Check sheet for the modelled part. Datum: model origin and axes. Units: mm. Face numbers are marked on the shaded views. A direction names the side the tool comes from. Give positions to 0.01 mm unless a question says otherwise; leave off trailing zeros. Write each loop counter-clockwise with the first axis right and the second up, starting at its lowest first coordinate (ties: lowest second). Pieces come first, ordered by that corner, then holes. Notation, with made-up numbers: M 51,79 L 81,79 A27 cw 81,110 Z; hole C -21,-19 d8. An arc over 180 degrees is marked long. Write item = value, one per line. Start each with the question number.
1) Sectioned sample at B-B, the plane x = 153. Record the cut outline in (y, z).
2) Sectioned sample at D-D, the plane z = 280. Record the cut outline in (x, y).
3) Sectioned sample at C-C, the plane x = -87. Record the cut outline in (y, z).
4) Scan lines: L1, parallel to Z at x = -26, y = -2.5; L2, parallel to Y at x = 56, z = 376; L3, parallel to X at y = 3.5, z = -16.5. Record each from-to range of solid material in increasing order.
5) Sectioned sample at A-A, the plane z = 67. Record the cut outline in (x, y).
6) Set-up check for the marked faces 1, 2 and 3: record each of +Z, -Z, +X, -X, +Y, -Y from which the full face is reachable in a straight line by a thin tool's end or side.
7) Gauge pin test, flat ends, axial feed: pin 1 (2 mm diameter, centred on x = -150.5, y = -1, fed in from -Z); pin 2 (6 mm diameter, centred on x = 18.5, z = 249.5, fed in from +Y); pin 3 (0.8 mm diameter, centred on x = 141.5, y = -0.5, fed in from +Z). Record the tip position at first contact, or that the pin passes through.
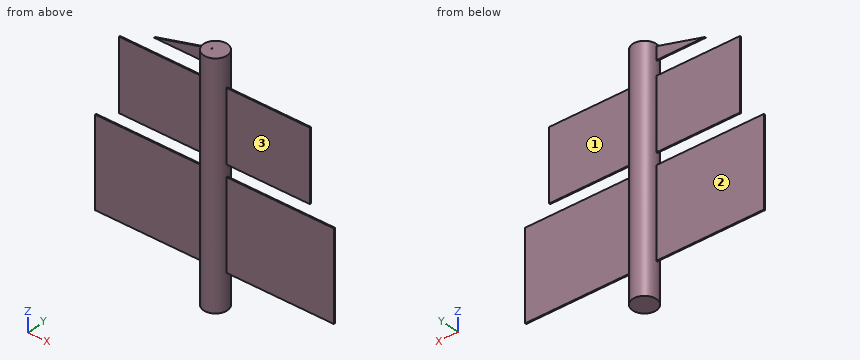
from build123d import *

# Parameters (mm, degrees)
F0_W     = 25.4
F0_H     = 508
F2_W     = 508
F2_H     = 190.5
F3_DEPTH = 2.54
F4_W     = 406.4
F4_H     = 152.4
F5_DEPTH = 2.54


with BuildPart() as f1:
    # F0 (on Front) → F1 (revolve)
    with BuildSketch(Plane.XZ):
        with Locations((12.7, 197.317208)):
            Rectangle(F0_W, F0_H)
    revolve(axis=Axis((0, 0, 197.317208), (0, 0, 1)))

    # F2 (on Front) → F3 (join)
    with BuildSketch(Plane.XZ):
        with Locations((0, 114.767208)):
            Rectangle(F2_W, F2_H)
    extrude(amount=F3_DEPTH)

    # F4 (on Front) → F5 (join)
    with BuildSketch(Plane.XZ):
        with Locations((0, 311.617208)):
            Rectangle(F4_W, F4_H)
        Polygon((-6.016195, 419.029802), (-6.016195, 452.049802), (-128.64849, 419.029802), align=None)
    extrude(amount=F5_DEPTH)


solid = f1.part
Data:
q1.outline = M -2.54,19.52 L 0,19.52 L 0,210.02 L -2.54,210.02 Z; M -2.54,235.42 L 0,235.42 L 0,387.82 L -2.54,387.82 Z
q2.outline = M -203.2,-2.54 L -25.27,-2.54 A25.4 ccw 25.27,-2.54 L 203.2,-2.54 L 203.2,0 L 25.4,0 A25.4 ccw -25.4,0 L -203.2,0 Z
q3.outline = M -2.54,19.52 L 0,19.52 L 0,210.02 L -2.54,210.02 Z; M -2.54,235.42 L 0,235.42 L 0,387.82 L -2.54,387.82 Z; M -2.54,419.03 L 0,419.03 L 0,430.24 L -2.54,430.24 Z
q4.L1 = 19.52 to 210.02, 235.42 to 387.82, 419.03 to 446.67
q4.L2 = -2.54 to 0
q4.L3 = -25.16 to 25.16
q5.outline = M -254,-2.54 L -25.27,-2.54 A25.4 ccw 25.27,-2.54 L 254,-2.54 L 254,0 L 25.4,0 A25.4 ccw -25.4,0 L -254,0 Z
q6.face_1 = +Z, -Z, +X, +Y
q6.face_2 = +Z, -Z, -X, +Y
q6.face_3 = +Z, -Z, +X, -Y
q7.pin_1 = 19.52
q7.pin_2 = 20.12
q7.pin_3 = 387.82
